The figure shows three views and two pictorial views of one solid part (mm, origin at its lowest corner). Answer the questions. A direction names the side the tool comes from. Coordinates: 2 decimals unless noted, no trailing zeros. Order: outer loops, then holes, each group sorted by start corner. A loop starts at its lowest first (then second) coordinate and runs counter-clockwise, first axis right, second up. Notation, with made-up numbers: (71.25, 58) -> (96.25, 58) arc R35 ccw to (96.25, 96) -> close; hole circle Ø1 at (-2.5, 84). An arc over 180 degrees is marked (long way). Return JSON: item names as keys, results as strings.
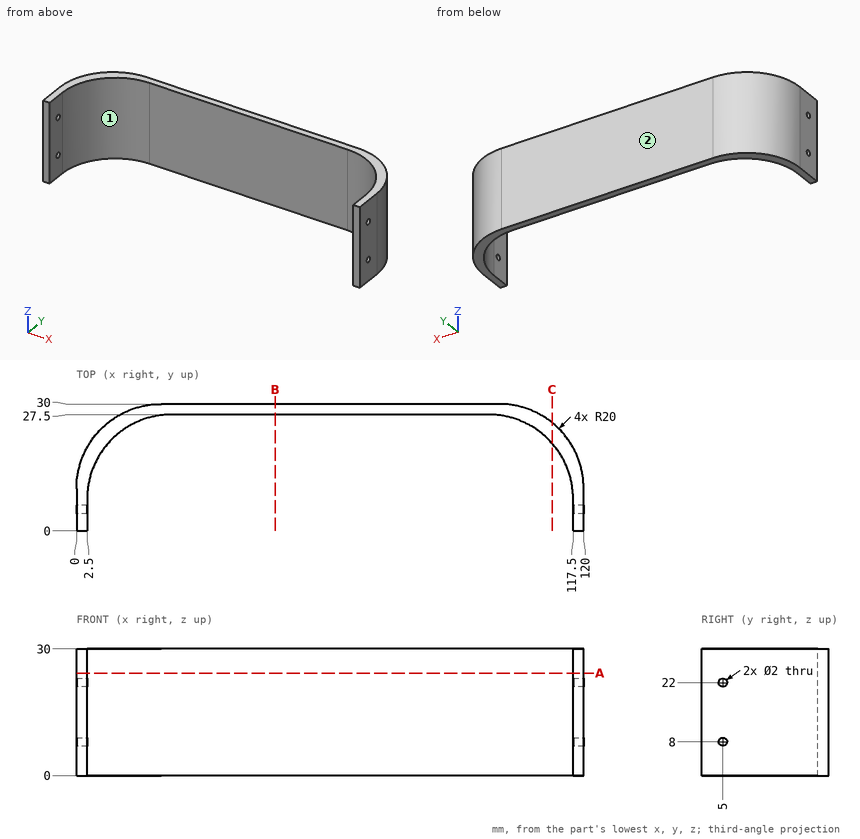
Item 1: The part is cut by section C-C on x = 112.5. Determine the outline of the cut face in (y, z).
Answer list:
{"outline": "(20.73, 0) -> (25.61, 0) -> (25.61, 30) -> (20.73, 30) -> close"}
Item 2: The part is cut by section B-B on x = 47. Determine the outline of the cut face in (y, z), plus the area to 3 significant figures.
Answer list:
{"outline": "(27.5, 0) -> (30, 0) -> (30, 30) -> (27.5, 30) -> close", "area": "75.0 mm2"}
Item 3: Find the intervals of material crossed by probe 1 along X at (y, z) = (6, 4.5); probe 2 along Y at (x, z) = (80, 24.25); probe 3 along X at (y, z) = (20, 22), in increasing order.
Answer list:
{"probe 1": "0 to 2.5, 117.5 to 120", "probe 2": "27.5 to 30", "probe 3": "2.68 to 6.89, 113.11 to 117.32"}
Item 4: The part is cut by section A-A on z = 24.25. Determine the outline of the cut face in (x, y), plus the area to 4 significant figures.
Answer list:
{"outline": "(0, 0) -> (2.5, 0) -> (2.5, 7.5) arc R20 cw to (22.5, 27.5) -> (97.5, 27.5) arc R20 cw to (117.5, 7.5) -> (117.5, 0) -> (120, 0) -> (120, 10) arc R20 ccw to (100, 30) -> (20, 30) arc R20 ccw to (0, 10) -> close", "area": "437.5 mm2"}
Item 5: Flat-ended cylindrical pins translate along their axes: pin 1 (1.2 mm diameter, centred on y = 5, z = 8, fed in from -X); pin 2 (1 mm diameter, centred on x = 83.5, z = 9, fed in from -Y); pin 3 (6 mm diameter, centred on y = 22.5, z = 25.5, fed in from -X). Find the tip coordinate at first contact, or state that the pin passes through.
Answer list:
{"pin 1": "through", "pin 2": "y = 27.5", "pin 3": "x = 2.4"}
Item 6: Which of the six approach directions +Z, -Z, +X, -X, +Y, -Y give full straight-line access (tool end or side, diameter ignored) to the marked faces 1 and 2?
Answer list:
{"face 1": "+Z, -Z, -Y", "face 2": "+Z, -Z, +X, -X, +Y"}
